Build history of the part. All positions in model axes, mm. A direction names the side the tool comes from. Give positions to 0.01 mm unless a question says otherwise; leave off trailing zeros. Loops run counter-clockwise (first coordinate to the right, second up) from the corner with the lowest first, then second, coordinate; pieces in that order, holes last.
1) Band-saw the part on C-C on y = -1.25. List the corners of the cut face in (x, z), then the cut area to 3 significant figures.
2) Band-saw the part on B-B on z = 7.75. List the corners of the cut face in (x, y), then the cut area to 3 significant figures.
3) 3-axis set-ups, long thin cutter, end or side, ignore diameter. For faces 1 (the flat face through (-1, -6, 1.968)), 2 (the flat face through (-0.63, -9.06, 3.55)), 3 (the flat face through (-0.63, -3.67, 3.5)), 4 (the flat face through (-1, -6, 8.192)), 5 (the flat face through (-0.63, -3.64, 6.61)): which of +Z, -Z, +X, -X, +Y, -Y reach the whole face in a straight line?
4) Flat gauge pins, fed straight in: P1, Ø1.5, axis at y = -5.5, z = 6, coming from the -X side; P2, Ø0.6, axis at x = -1, y = -6, coming from the +Z side. Where does each tip first touch, or does it go through?
5) Two-plate mould, pull along Z, no slides. Class faces 6 (the flat face through (13, -6, 10.16)), 7 (the flat face through (-1.27, -9, 6)), 8 (the flat face through (-0.626, -4.324, 3.889)): +Z half, -Z half, draft (parallel to the pull), parting line (faces both ways), or undercut.
6) Wall check: line 1 (X direction, y = -5.5, z = 1.5). Give the ranges that are in metal, low to high.
7) Band-saw the part on A-A on y = -5.75. List the corners of the cut face in (x, z).
8) Band-saw the part on D-D on z = 1.5. List the corners of the cut face in (x, y), then the cut area to 3 significant figures.
```python
from build123d import *

# Parameters (mm, degrees)
SKETCH1_W           = 25.4
SKETCH1_H           = 12.7
BOSS_EXTRUDE1_DEPTH = 10.16
BOSS_EXTRUDE2_DEPTH = 1.27


with BuildPart() as part:
    # Sketch1 → Boss-Extrude1 (new body)
    with BuildSketch(Plane.XY):
        with Locations((12.7, -6.35)):
            Rectangle(SKETCH1_W, SKETCH1_H)
    extrude(amount=BOSS_EXTRUDE1_DEPTH)

    # Sketch2 → Boss-Extrude2 (add)
    with BuildSketch(Plane.ZY):
        Polygon((5.08, -2.756658991), (8.191924598, -4.553329495), (8.191924598, -8.146670505), (5.08, -9.943341009), (1.968075402, -8.146670505), (1.968075402, -4.553329495), align=None)
        Polygon((7.429924598, -4.993270401), (7.429924598, -7.706729599), (5.08, -9.063459199), (2.730075402, -7.706729599), (2.730075402, -4.993270401), (5.08, -3.636540801), align=None, mode=Mode.SUBTRACT)
    extrude(amount=BOSS_EXTRUDE2_DEPTH)


solid = part.part
```
Findings below:
1. outline: (0, 0) - (25.4, 0) - (25.4, 10.16) - (0, 10.16) - close
1. area: 258 mm2
2. outline: (-1.27, -8.4) - (0, -8.4) - (0, -12.7) - (25.4, -12.7) - (25.4, 0) - (0, 0) - (0, -4.3) - (-1.27, -4.3) - close
2. area: 328 mm2
3. face 1: -Z, -X, +Y, -Y
3. face 2: -Z, -X, -Y
3. face 3: -Z, -X, +Y
3. face 4: +Z, -X, +Y, -Y
3. face 5: +Z, -X, +Y
4. P1: stops at x = 0
4. P2: stops at z = 8.19
5. face 6: +Z half
5. face 7: draft
5. face 8: undercut
6. line 1: x = 0 to 25.4
7. outline: (-1.27, 1.97) - (0, 1.97) - (0, 0) - (25.4, 0) - (25.4, 10.16) - (0, 10.16) - (0, 8.19) - (-1.27, 8.19) - (-1.27, 7.43) - (0, 7.43) - (0, 2.73) - (-1.27, 2.73) - close
8. outline: (0, -12.7) - (25.4, -12.7) - (25.4, 0) - (0, 0) - close
8. area: 323 mm2
